Read the model definition and answer for the solid it produces. Units are mm, in the model's axes. A direction names the side the tool comes from. Round coordinates to 2 decimals unless told otherwise and drop trailing zeros. Order: outer loops, then holes, each group sorted by start corner. A loop starts at its lowest first (then second) coordinate and runs counter-clockwise, first axis right, second up. Notation, with made-up numbers: (-2, 38.25) - (39, 38.25) arc R33 ccw to (39, 73.25) - close; hole circle Ø11 at (-22.75, 56). An arc over 180 degrees is marked (long way). Put each result on its own line as item: value. Start each with the question number.
Q1. Section A-A on y = -5 is taken. Give the vertices of the cut face in (x, z).
Q2. Section D-D on y = 3 is taken. Give the vertices of the cut face in (x, z), then the cut area to 3 significant figures.
Q3. Section C-C on x = 0 is taken. Give the vertices of the cut face in (y, z), then the cut area to 3 significant figures.
Q4. Section B-B on z = 6.5 is taken. Give the vertices of the cut face in (x, y).
Q5. Each of these flat-tipped pins is pushed along its axis until it touches: pin 1 Ø6 at (y, z) = (7, 13) entering from -X; pin 2 Ø9 at (x, z) = (-9, 8.5) entering from -Y; pin 3 Ø5 at (y, z) = (13, 9) entering from +X. Where does it stop, or does it pass through?
Q6. Which of the six approach directions +Z, -Z, +X, -X, +Y, -Y give full straight-line access (tool end or side, diameter ignored) to faces 5 (the face through (0, -11, 1.2)), 6 (the face through (-43, 23, 0.2)), 7 (the face through (2, 0, 0)), 8 (the face through (-43, -23, 0.2))?
Q7. For a pull along Y with two mould halves and no side action, classify faces 1 (the face through (1, -21, 11)), 2 (the face through (43, -24, 0.2)), 3 (the face through (1, 22.2, 10)), 4 (the face through (0, -0.603, 11)) as pulls with the +Y half, pulls with the -Y half, needs draft (parallel to the pull), parting line crosses it, or undercut.
Q8. Find the intervals of material crossed by line 1 along Y through (x, z) = (31, 12.5); line 2 along X through (y, z) = (18, 11.25); line 3 along X through (y, z) = (-20, 18.25), in increasing order. Write a range as from..to.
from build123d import *

# Parameters (mm, degrees)
SKETCH_1_W          = 86
SKETCH_1_H          = 44.4
EXTRUDE_1_DEPTH     = 19.6
EXTRUDE_2_DEPTH     = 5
SKETCH_3_W          = 83.2
SKETCH_3_H          = 20.402884615
SKETCH_3_H_2        = 20.397115385
CUT_EXTRUDE_1_DEPTH = 18.4
FILLET_1_R          = 3
EXTRUDE_3_DEPTH     = 0.2


with BuildPart() as part:
    # Эскиз1 → Бобышка-Вытянуть1 (new body)
    with BuildSketch(Plane.XY):
        Rectangle(SKETCH_1_W, SKETCH_1_H)
    extrude(amount=EXTRUDE_1_DEPTH)

    # Эскиз2 → Бобышка-Вытянуть2 (add)
    with BuildSketch(Plane.XY):
        with BuildLine():
            Line((43, 17.2), (43, 13.108775687))
            ThreePointArc((43, 13.108775687), (53.273546839, 0), (43, -13.108775687))
            Line((43, -13.108775687), (43, -17.2))
            ThreePointArc((43, -17.2), (57.273546839, 0), (43, 17.2))
        make_face()
    extrude(amount=EXTRUDE_2_DEPTH)

    # Эскиз3 → Вырез-Вытянуть1 (cut)
    with BuildSketch(Plane.XY.offset(19.6)):
        with Locations((0.2, 10.798557692)):
            Rectangle(SKETCH_3_W, SKETCH_3_H)
        with Locations((0.2, -10.801442308)):
            Rectangle(SKETCH_3_W, SKETCH_3_H_2)
    extrude(amount=-CUT_EXTRUDE_1_DEPTH, mode=Mode.SUBTRACT)

    # Скругление1
    fillet_1_edges = [part.edges().sort_by_distance(p)[0] for p in [
        (-41.4, 21, 10.4),
        (-41.4, -21, 10.4),
        (-43, -22.2, 9.8),
        (-43, 22.2, 9.8),
    ]]
    fillet(fillet_1_edges, radius=FILLET_1_R)

    # Эскиз4 → Бобышка-Вытянуть3 (add)
    with BuildSketch(Plane(origin=(0, 0, 0), x_dir=(-1, 0, 0), z_dir=(0, 0, -1))):
        with BuildLine():
            Line((-49.68910779, 14.419835333), (-30.736733343, 22.2))
            ThreePointArc((-30.736733343, 22.2), (-45.063461681, 30.125769311), (-49.68910779, 14.419835333))
        make_face()
        with BuildLine():
            Line((43, 10.144768059), (30.517095223, 22.2))
            ThreePointArc((30.517095223, 22.2), (48.148575221, 27.966485606), (43, 10.144768059))
        make_face()
        with BuildLine():
            Line((43, -10.144768059), (30.517095223, -22.2))
            ThreePointArc((30.517095223, -22.2), (48.148575221, -27.966485606), (43, -10.144768059))
        make_face()
        with BuildLine():
            Line((-49.68910779, -14.419835333), (-30.736733343, -22.2))
            ThreePointArc((-30.736733343, -22.2), (-45.063461681, -30.125769311), (-49.68910779, -14.419835333))
        make_face()
    extrude(amount=-EXTRUDE_3_DEPTH)


solid = part.part
Findings:
1. outline: (-43, 0) - (43, 0) - (43, 19.6) - (41.8, 19.6) - (41.8, 1.2) - (-41.4, 1.2) - (-41.4, 19.6) - (-43, 19.6) - close; (52.31, 0) - (56.54, 0) - (56.54, 5) - (52.31, 5) - close
2. outline: (-43, 0) - (43, 0) - (43, 19.6) - (41.8, 19.6) - (41.8, 1.2) - (-41.4, 1.2) - (-41.4, 19.6) - (-43, 19.6) - close; (52.94, 0) - (57.01, 0) - (57.01, 5) - (52.94, 5) - close
2. area: 175 mm2
3. outline: (-22.2, 0) - (22.2, 0) - (22.2, 19.6) - (21, 19.6) - (21, 1.2) - (0.6, 1.2) - (0.6, 19.6) - (-0.6, 19.6) - (-0.6, 1.2) - (-21, 1.2) - (-21, 19.6) - (-22.2, 19.6) - close
3. area: 120 mm2
4. outline: (-43, -19.2) arc R3 ccw to (-40, -22.2) - (43, -22.2) - (43, 22.2) - (-40, 22.2) arc R3 ccw to (-43, 19.2) - close; hole (-41.4, -18) arc R3 ccw to (-38.4, -21) - (41.8, -21) - (41.8, -0.6) - (-41.4, -0.6) - close; hole (-41.4, 0.6) - (41.8, 0.6) - (41.8, 21) - (-38.4, 21) arc R3 ccw to (-41.4, 18) - close
5. pin 1: x = -43
5. pin 2: y = -22.2
5. pin 3: x = 43
6. face 5: +Z
6. face 6: +Z, -X, +Y
6. face 7: -Z, +X, -X, +Y, -Y
6. face 8: +Z, -X, -Y
7. face 1: undercut
7. face 2: needs draft
7. face 3: pulls with the +Y half
7. face 4: undercut
8. line 1: -22.2..-21, -0.6..0.6, 21..22.2
8. line 2: -43..-41.4, 41.8..43
8. line 3: -42.89..-40.64, 41.8..43
